from build123d import *
from build123d.topology import SkipClean

# Parameters (mm, degrees)
SKETCH1_R           = 120.65
BOSS_EXTRUDE1_DEPTH = 63.5
SKETCH2_R           = 116.84
CUT_EXTRUDE1_DEPTH  = 50.8
BOSS_EXTRUDE3_START = 12.7
SKETCH4_R           = 120.65
BOSS_EXTRUDE3_DEPTH = 12.7
SKETCH5_R           = 144.351080184
BOSS_EXTRUDE4_DEPTH = 12.7
SKETCH6_R           = 152.4
BOSS_EXTRUDE5_DEPTH = 50.8
SKETCH8_W           = 330.2
SKETCH8_H           = 330.2
BOSS_EXTRUDE6_DEPTH = 12.7
SKETCH7_R           = 6.35
CUT_EXTRUDE2_DEPTH  = 250.838407776


with BuildPart() as part:
    # Sketch1 → Boss-Extrude1 (new body)
    with BuildSketch(Plane(origin=(0, 0, 0), x_dir=(1, 0, 0), z_dir=(0, 1, 0))):
        with Locations(Location((0, 0, 0), (0, 0, 270))):
            Circle(SKETCH1_R)
    extrude(amount=BOSS_EXTRUDE1_DEPTH)

    # Sketch2 → Cut-Extrude1 (cut)
    with BuildSketch(Plane(origin=(0, 63.5, 0), x_dir=(1, 0, 0), z_dir=(0, 1, 0))):
        with Locations(Location((0, 0, 0), (0, 0, 270))):
            Circle(SKETCH2_R)
    extrude(amount=-CUT_EXTRUDE1_DEPTH, mode=Mode.SUBTRACT)

    # Sketch4 → Boss-Extrude3 (add)
    with BuildSketch(Plane.XZ.offset(BOSS_EXTRUDE3_START)):
        with BuildLine():
            ThreePointArc((-119.58085221, -16.026299781), (-120.65, 0), (-119.58085221, 16.026299781))
            Line((-119.58085221, 16.026299781), (-128.324780403, 16.026299781))
            ThreePointArc((-128.324780403, 16.026299781), (-144.351080184, 0), (-128.324780403, -16.026299781))
            Line((-128.324780403, -16.026299781), (-119.58085221, -16.026299781))
        make_face()
        with BuildLine():
            Line((-16.026299781, 128.324780403), (-16.026299781, 119.58085221))
            ThreePointArc((-16.026299781, 119.58085221), (0, 120.65), (16.026299781, 119.58085221))
            Line((16.026299781, 119.58085221), (16.026299781, 128.324780403))
            ThreePointArc((16.026299781, 128.324780403), (0, 144.351080184), (-16.026299781, 128.324780403))
        make_face()
        with Locations(Location((0, 0, 0), (0, 0, 277.633330587))):
            Circle(SKETCH4_R)
        with BuildLine():
            Line((128.324780403, 16.026299781), (119.58085221, 16.026299781))
            ThreePointArc((119.58085221, 16.026299781), (120.382416322, 8.030961363), (120.65, 0))
            ThreePointArc((120.65, 0), (120.382416322, -8.030961363), (119.58085221, -16.026299781))
            Line((119.58085221, -16.026299781), (128.324780403, -16.026299781))
            ThreePointArc((128.324780403, -16.026299781), (144.351080184, 0), (128.324780403, 16.026299781))
        make_face()
        with BuildLine():
            ThreePointArc((16.026299781, -119.58085221), (0, -120.65), (-16.026299781, -119.58085221))
            Line((-16.026299781, -119.58085221), (-16.026299781, -128.324780403))
            ThreePointArc((-16.026299781, -128.324780403), (0, -144.351080184), (16.026299781, -128.324780403))
            Line((16.026299781, -128.324780403), (16.026299781, -119.58085221))
        make_face()
    extrude(amount=-BOSS_EXTRUDE3_DEPTH)

    # Sketch5 → Boss-Extrude4 (add)
    with SkipClean():  # the faces are left unmerged after this step: merging them gives an invalid solid
        with BuildSketch(Plane.XZ.offset(12.7)):
            with Locations(Location((0, 0, 0), (0, 0, 270))):
                Circle(SKETCH5_R)
        extrude(amount=BOSS_EXTRUDE4_DEPTH)
    add(part.part.scale(1), mode=Mode.REPLACE)  # the faces are merged on a copy

    # Sketch6 → Boss-Extrude5 (add)
    with BuildSketch(Plane.XZ.offset(25.4)):
        with Locations(Location((0, 0, 0), (0, 0, 270))):
            Circle(SKETCH6_R)
    extrude(amount=BOSS_EXTRUDE5_DEPTH)

    # Sketch8 → Boss-Extrude6 (add)
    with BuildSketch(Plane.XZ.offset(76.2)):
        Rectangle(SKETCH8_W, SKETCH8_H)
    extrude(amount=BOSS_EXTRUDE6_DEPTH)

    # Sketch7 → Cut-Extrude2 (cut, through all)
    with BuildSketch(Plane(origin=(0, 0, 0), x_dir=(1, 0, 0), z_dir=(0, 1, 0))):
        with Locations(Location((0, 128.324780403, 0), (0, 0, 270))):
            Circle(SKETCH7_R)
        with Locations(Location((-128.324780403, 0, 0), (0, 0, 270))):
            Circle(SKETCH7_R)
        with Locations(Location((0, -128.324780403, 0), (0, 0, 270))):
            Circle(SKETCH7_R)
        with Locations(Location((128.324780403, 0, 0), (0, 0, 270))):
            Circle(SKETCH7_R)
    extrude(amount=-CUT_EXTRUDE2_DEPTH, mode=Mode.SUBTRACT)


solid = part.part
CAD build for the part. Positions are in the model's coordinates, mm. A direction names the side the tool comes from. Round coordinates to 2 decimals unless told otherwise and drop trailing zeros. Order: outer loops, then holes, each group sorted by start corner. A loop starts at its lowest first (then second) coordinate and runs counter-clockwise, first axis right, second up. Notation, with made-up numbers: (16.5, 78) -> (69.5, 78) arc R35 cw to (69.5, 115) -> close; hole circle Ø1 at (-31.5, -25.75). An arc over 180 degrees is marked (long way). Write item = value, one per line. Start each with the question number.
(1) Probe line 1 (X direction, y = -66.5, z = 0); line 2 (Y direction, x = 94, z = 43.5); line 3 (Y direction, x = 149, z = -31.5). List the from-to ranges inside material, lowest first. Write a range as [from, to].
(2) Pull direction X, two halves, no side cores. Call faces 5 (the cylindrical face through (-134.524, -43.828, -1.377)), 6 (the flat face through (-74, -76.2, -134)), 7 (the cylindrical face through (-144.347, -6.439, 0.352)), 8 (the cylindrical face through (0.28, -43.83, 121.98)): released by +X, released by -X, zero draft, split by the parting line, or undercut.
(3) Which spindle directions (+Z, -Z, +X, -X, +Y, -Y) get a long thin tool onto all of the face, cutting with end or side? Do faces 1 (the cylindrical face through (144.347, -6.439, -0.352)), 2 (the flat face through (124, -6, -16.026)), 3 (the flat face through (-124, -6, 16.026)), 4 (the flat face through (124, -6, 16.026)). Say none if no direction does.
(4) Cut at A-A, the plane y = -61. List the corners of the cut face in (x, z).
(5) Cut at B-B, the plane z = -32. List the corners of the cut face in (x, y).
(6) Pin check, flat tips, straight feed: P1, Ø2.5, axis at y = -4, z = 124.5, coming from the -X side; P2, Ø12, axis at y = -9.5, z = 21, coming from the +X side; P3, Ø7, axis at x = -125.5, y = -5, coming from the +Z side. Stop position of each tip, or through.
(7) Cut at D-D, the plane y = 40. List the corners of the cut face in (x, z).
Model answer:
q1.line_1 = [-152.4, -134.67], [-121.97, 121.97], [134.67, 152.4]
q1.line_2 = [-88.9, 12.7]
q1.line_3 = [-88.9, -25.4]
q2.face_5 = undercut
q2.face_6 = zero draft
q2.face_7 = released by -X
q2.face_8 = undercut
q3.face_1 = +X, +Y
q3.face_2 = -Z, +X, +Y
q3.face_3 = +Z, -X, +Y
q3.face_4 = +Z, +X, +Y
q4.outline = circle Ø304.8 at (0, 0); hole circle Ø12.7 at (-128.32, 0); hole circle Ø12.7 at (0, -128.32); hole circle Ø12.7 at (0, 128.32); hole circle Ø12.7 at (128.32, 0)
q5.outline = (-165.1, -88.9) -> (165.1, -88.9) -> (165.1, -76.2) -> (149, -76.2) -> (149, -25.4) -> (140.76, -25.4) -> (140.76, -12.7) -> (116.33, -12.7) -> (116.33, 63.5) -> (112.37, 63.5) -> (112.37, 12.7) -> (-112.37, 12.7) -> (-112.37, 63.5) -> (-116.33, 63.5) -> (-116.33, -12.7) -> (-140.76, -12.7) -> (-140.76, -25.4) -> (-149, -25.4) -> (-149, -76.2) -> (-165.1, -76.2) -> close
q6.P1 = -16.03
q6.P2 = 143.47
q6.P3 = 16.03
q7.outline = circle Ø241.3 at (0, 0); hole circle Ø233.68 at (0, 0)
